```python
from build123d import *

# Parameters (mm, degrees)
F0_R     = 125
F0_R_2   = 9
F0_R_3   = 70.75
F0_R_4   = 69.85
F1_DEPTH = 22
F3_R     = 100
F3_R_2   = 9
F3_R_3   = 45.25
F3_R_4   = 44.45
F4_DEPTH = 20


with BuildPart() as f1:
    # F0 (on Right) → F1 (new body)
    with BuildSketch(Plane.YZ):
        Circle(F0_R)
        with Locations((-74.246212, -74.246212)):
            Circle(F0_R_2, mode=Mode.SUBTRACT)
        with Locations((0, -105)):
            Circle(F0_R_2, mode=Mode.SUBTRACT)
        with Locations((74.246212, -74.246212)):
            Circle(F0_R_2, mode=Mode.SUBTRACT)
        with Locations((-105, 0)):
            Circle(F0_R_2, mode=Mode.SUBTRACT)
        with Locations((-74.246212, 74.246212)):
            Circle(F0_R_2, mode=Mode.SUBTRACT)
        Circle(F0_R_3, mode=Mode.SUBTRACT)
        with Locations((105, 0)):
            Circle(F0_R_2, mode=Mode.SUBTRACT)
        with Locations((0, 105)):
            Circle(F0_R_2, mode=Mode.SUBTRACT)
        with Locations((74.246212, 74.246212)):
            Circle(F0_R_2, mode=Mode.SUBTRACT)
        Circle(F0_R_3)
        Circle(F0_R_4, mode=Mode.SUBTRACT)
    extrude(amount=F1_DEPTH)



with BuildPart() as f4:
    # F3 (on offset) → F4 (new body)
    with BuildSketch(Plane.YZ.offset(100)):
        Circle(F3_R)
        with Locations((-56.568542, -56.568542)):
            Circle(F3_R_2, mode=Mode.SUBTRACT)
        with Locations((0, -80)):
            Circle(F3_R_2, mode=Mode.SUBTRACT)
        with Locations((56.568542, -56.568542)):
            Circle(F3_R_2, mode=Mode.SUBTRACT)
        with Locations((-80, 0)):
            Circle(F3_R_2, mode=Mode.SUBTRACT)
        with Locations((-56.568542, 56.568542)):
            Circle(F3_R_2, mode=Mode.SUBTRACT)
        Circle(F3_R_3, mode=Mode.SUBTRACT)
        with Locations((80, 0)):
            Circle(F3_R_2, mode=Mode.SUBTRACT)
        with Locations((0, 80)):
            Circle(F3_R_2, mode=Mode.SUBTRACT)
        with Locations((56.568542, 56.568542)):
            Circle(F3_R_2, mode=Mode.SUBTRACT)
        Circle(F3_R_3)
        Circle(F3_R_4, mode=Mode.SUBTRACT)
    extrude(amount=F4_DEPTH)


with BuildPart() as f1_1:
    add(f1.part)

    add(f4.part)  # F7 merges F4
    # F6 (on Front) → F7 (revolve)
    with BuildSketch(Plane.XZ):
        Polygon((100, 45.25), (22, 70.75), (22, 69.85), (100, 44.45), align=None)
    revolve(axis=Axis((82.332404, 0, 0), (1, 0, 0)))


solid = f1_1.part
```
The listing builds one solid part. Answer for the finished solid, in the listing's coordinates (mm). A direction names the side the tool comes from. Give positions to 0.01 mm unless a question says otherwise; leave off trailing zeros. Order: outer loops, then holes, each group sorted by start corner. A loop starts at its lowest first (then second) coordinate and runs counter-clockwise, first axis right, second up. Notation, with made-up numbers: (85, -25) - (100, -25) arc R15 cw to (100, -9) - close; hole circle Ø6 at (30.5, 15). An arc over 180 degrees is marked (long way). Answer in a Markdown table with one row per item. Add a question column.
Q1. The part is cut by section A-A (y = -103.5). Determine the outline of the cut face in (x, z), then the cut area to 3 significant figures.
Q2. The part is cut by section B-B (z = 80). Determine the outline of the cut face in (x, y).
Q3. Given P1, Ø4, axis at y = 93.5, z = -18.5, coming from the -X side; P2, Ø16, axis at y = -105, z = 0, coming from the -X side; P3, Ø2, axis at x = 65.5, z = 31.5, coming from the -Y side; P4, Ø6, axis at x = 106.5, z = 58.5, coming from the -Y side, each flat-ended and moving along its own axis, determine where each tip first touches the part or whether it passes through.
Q4. The part is cut by section D-D (z = 105). Determine the outline of the cut face in (x, y), then the cut area to 3 significant figures.
Q5. For a pull along Y with two mould halves and no side action, classify faces 1 (the cylindrical face through (10.846, -70.093, 66.262)), 2 (the cylindrical face through (10.85, -70.09, -82.23)), 3 (the flat face through (100, -1, 46)), 4 (the cylindrical face through (10.85, -124.88, 5.5)) as released by +Y, released by -Y, zero draft, split by the parting line, or undercut.
Q6. Which of the six approach directions +Z, -Z, +X, -X, +Y, -Y give full straight-line access (tool end or side, diameter ignored) to faces 5 (the cylindrical face through (10.846, -1.951, -113.786)), 6 (the flat face through (120, -1, 46)), 7 (the cylindrical face through (109.86, -48.255, 53.121))?
Q7. Find the intervals of material crossed by line 1 along Z through (x, y) = (113.5, 0); line 2 along Z through (x, y) = (6, 0); line 3 along X through (y, z) = (-76.5, -36.5), in increasing order. Write a range as [from, to].
Determined:
| question | item | result |
|---|---|---|
| 1 | outline | (0, -70.09) - (22, -70.09) - (22, -8.87) - (0, -8.87) - close; (0, 8.87) - (22, 8.87) - (22, 70.09) - (0, 70.09) - close |
| 1 | area | 2,690 mm² |
| 2 | outline | (0, -96.05) - (22, -96.05) - (22, -81.17) - (0, -81.17) - close; (0, -67.33) - (22, -67.33) - (22, 67.33) - (0, 67.33) - close; (0, 81.17) - (22, 81.17) - (22, 96.05) - (0, 96.05) - close; (100, -60) - (120, -60) - (120, -9) - (100, -9) - close; (100, 9) - (120, 9) - (120, 60) - (100, 60) - close |
| 3 | P1 | stops at x = 0 |
| 3 | P2 | stops at x = 100 |
| 3 | P3 | stops at y = -47.7 |
| 3 | P4 | stops at y = -83.19 |
| 4 | outline | (0, -67.82) - (22, -67.82) - (22, -9) - (0, -9) - close; (0, 9) - (22, 9) - (22, 67.82) - (0, 67.82) - close |
| 4 | area | 2,590 mm² |
| 5 | face 1 | undercut |
| 5 | face 2 | undercut |
| 5 | face 3 | zero draft |
| 5 | face 4 | split by the parting line |
| 6 | face 5 | -X |
| 6 | face 6 | +Z, -Z, +X, +Y, -Y |
| 6 | face 7 | +X |
| 7 | line 1 | z = [-100, -89], [-71, -44.45], [44.45, 71], [89, 100] |
| 7 | line 2 | z = [-125, -114], [-96, -69.85], [69.85, 96], [114, 125] |
| 7 | line 3 | x = [0, 22], [100, 120] |
